Read the model definition and answer for the solid it produces. Units are mm, in the model's axes. Coordinates: 2 decimals unless noted, no trailing zeros. Order: outer loops, then holes, each group sorted by start corner. A loop starts at its lowest first (then second) coordinate and runs counter-clockwise, first axis right, second up.
Autodesk Inventor part; units mm, degrees
ref_plane "YZ Plane" through (0, 0, 0) normal (1, 0, 0) x (0, 1, 0)
ref_plane "XZ Plane" through (0, 0, 0) normal (0, 1, 0) x (-1, 0, 0)
ref_plane "XY Plane" through (0, 0, 0) normal (0, 0, 1) x (1, 0, 0)
sketch "Boceto1" plane through (0, 0, 0) normal (0, 0, 1) x (1, 0, 0)
  line L0 (0, 0) -> (50, 0)
  line L1 (50, 0) -> (50, 120)
  line L2 (50, 120) -> (0, 120)
  line L3 (0, 120) -> (0, 0)
  dimension "d0" = 50
  dimension "d1" = 120
extrude "Extrusión1" add sketch "Boceto1" along normal blind 6.4
sketch "Boceto2" plane through (0, 0, 6.4) normal (0, 0, 1) x (1, 0, 0)
  line L0 (50, 120) -> (0, 120)
  line L1 (25, 120) -> (25, 117)
  line L2 (25, 117) -> (25, 107.5)
  circle A0 centre (25, 107.5) radius 8
  point P0 (0, 0)
  dimension "d4" = 3
  dimension "d5" = 9.5
  dimension "d6" = 16
extrude "Extrusión2" cut sketch "Boceto2" against normal through all
properties part number "Base_cortadora"
1) Straight lines are drawn through the part: line 1 (Y direction, x = 25, z = 3.5); line 2 (X direction, y = 107.5, z = 2.5); line 3 (Y direction, x = 27, z = 5). For each, find the intervals that lie inside material, in ascending order.
A:
line 1: y = 0 to 99.5, 115.5 to 120
line 2: x = 0 to 17, 33 to 50
line 3: y = 0 to 99.75, 115.25 to 120
2) A cutting plane is placed at B-B, the plane x = 25. Determine the outline of the cut face in (y, z).
A:
outline: (0, 0) - (99.5, 0) - (99.5, 6.4) - (0, 6.4) - close; (115.5, 0) - (120, 0) - (120, 6.4) - (115.5, 6.4) - close
3) A cutting plane is placed at C-C, the plane z = 3.25. Determine the outline of the cut face in (x, y).
A:
outline: (0, 0) - (50, 0) - (50, 120) - (0, 120) - close; hole circle Ø16 at (25, 107.5)
4) A flat-ended cylindrical pin translates along its axis: pin 1 Ø6 at (x, y) = (12, 104.5) entering from -Z. Find the tip coordinate at first contact, or state that the pin passes through.
A:
pin 1: stops at z = 0
5) Determine the mould class of faces 1 (the flat face through (25, 61, 0)), 2 (the flat face through (25, 120, 3)), 3 (the cylindrical face through (23.27, 99.69, 3.24)) for opening direction Y: pulls with the +Y half, pulls with the -Y half, needs draft (parallel to the pull), parting line crosses it, or undercut.
A:
face 1: needs draft
face 2: pulls with the +Y half
face 3: undercut
6) A cutting plane is placed at A-A, the plane y = 107.5. Determine the outline of the cut face in (x, z), and give its area (3 significant figures).
A:
outline: (0, 0) - (17, 0) - (17, 6.4) - (0, 6.4) - close; (33, 0) - (50, 0) - (50, 6.4) - (33, 6.4) - close
area: 218 mm2
